from build123d import *

# Parameters (mm, degrees)
SKETCH_W     = 17.5
SKETCH_H     = 16.5
PAD_DEPTH    = 4
SKETCH002_W  = 14.5
SKETCH002_H  = 13.5
POCKET_DEPTH = 5
SKETCH003_W  = 1
SKETCH003_H  = 2.9
PAD001_DEPTH = 3
FILLET_R     = 1
FILLET001_R  = 2
CHAMFER_SIZE = 1


with BuildPart() as part:
    # Sketch → Pad (new body)
    with BuildSketch(Plane.XY):
        Rectangle(SKETCH_W, SKETCH_H)
    extrude(amount=PAD_DEPTH)

    # Sketch002 → Pocket (cut)
    with BuildSketch(Plane.XY.offset(3)):
        Rectangle(SKETCH002_W, SKETCH002_H)
    extrude(amount=POCKET_DEPTH, mode=Mode.SUBTRACT)

    # Sketch003 (on Face11 of Pocket) → Pad001 (join)
    with BuildSketch(Plane.XY.offset(3)):
        with Locations((-2.75, 0)):
            Rectangle(SKETCH003_W, SKETCH003_H)
        with Locations((2.75, 0)):
            Rectangle(SKETCH003_W, SKETCH003_H)
    extrude(amount=PAD001_DEPTH)

    # Fillet
    fillet_edges = [part.edges().sort_by_distance(p)[0] for p in [
        (2.75, 1.45, 3),
        (3.25, 0, 3),
        (2.75, -1.45, 3),
        (2.25, 0, 3),
        (-2.75, 1.45, 3),
        (-3.25, 0, 3),
        (-2.75, -1.45, 3),
        (-2.25, 0, 3),
    ]]
    fillet(fillet_edges, radius=FILLET_R)

    # Fillet001
    fillet001_edges = [part.edges().sort_by_distance(p)[0] for p in [
        (-8.75, 8.25, 2),
        (8.75, 8.25, 2),
        (8.75, -8.25, 2),
        (-8.75, -8.25, 2),
    ]]
    fillet(fillet001_edges, radius=FILLET001_R)

    # Chamfer
    chamfer_edges = [part.edges().sort_by_distance(p)[0] for p in [
        (-8.75, 0, 0),
        (-8.164214, 7.664214, 0),
        (-8.164214, -7.664214, 0),
        (0, 8.25, 0),
        (0, -8.25, 0),
        (8.164214, 7.664214, 0),
        (8.164214, -7.664214, 0),
        (8.75, 0, 0),
    ]]
    chamfer(chamfer_edges, length=CHAMFER_SIZE)


solid = part.part
CAD build for the part. Positions are in the model's coordinates, mm. A direction names the side the tool comes from. Round coordinates to 2 decimals unless told otherwise and drop trailing zeros. Write each loop counter-clockwise with the first axis right and the second up, starting at its lowest first coordinate (ties: lowest second). Pieces come first, ordered by that corner, then holes. Notation, with made-up numbers: M -4,84.25 L 49,84.25 A22 ccw 49,119.25 Z; hole C 4.5,-10.75 d5. An arc over 180 degrees is marked long. Put each result on its own line as item: value. Start each with the question number.
1) Saw through at A-A, the plane x = -0.75. Write the cut outline in (y, z), and give its area (3 significant figures).
2) Saw through at D-D, the plane y = -2.75. Write the cut outline in (x, z), and give its area (3 significant figures).
3) Pull direction Y, two halves, no side cores. Call faces 1 (the flat face through (2.25, 0, 5)), 2 (the cylindrical face through (2.77, 1.89, 3.17)), 3 (the flat face through (-0.09, 7.74, 0.49)): pulls with the +Y half, pulls with the -Y half, needs draft (parallel to the pull), parting line crosses it, or undercut.
4) Saw through at C-C, the plane x = 3. Write the cut outline in (y, z).
5) Pin check, flat tips, straight feed: pin 1 Ø1 at (y, z) = (0.5, 5) entering from -X; pin 2 Ø0.8 at (x, z) = (3, 5) entering from -Y; pin 3 Ø1 at (y, z) = (0, 5.5) entering from +X. Stop position of each tip, or through.
6) Saw through at B-B, the plane y = 0.25. Write the cut outline in (x, z).
7) 3-axis set-ups, long thin cutter, end or side, ignore diameter. For faces 4 (the flat face through (-3, 1.45, 5)), 5 (the flat face through (3, -1.45, 5)), 6 (the conical face through (7.716, 7.238, 0.382)), 7 (the cylindrical face through (-2.73, 1.89, 3.17)), 8 (the flat face through (-2.25, 0, 5)): which of +Z, -Z, +X, -X, +Y, -Y reach the whole face in a straight line?
8) Drill centre lines: probe 1 along Y at (x, z) = (-3, 3.9); probe 2 along Y at (x, z) = (-0.5, 3.6); probe 3 along Z at (x, y) = (5.25, 5.75). Where is each one in solid material? Low to high. Write a range as [from, to].
Resolved:
1. outline: M -8.25,1 L -7.25,0 L 7.25,0 L 8.25,1 L 8.25,4 L 6.75,4 L 6.75,3 L -6.75,3 L -6.75,4 L -8.25,4 Z
1. area: 51.5 mm²
2. outline: M -8.75,1 L -7.75,0 L 7.75,0 L 8.75,1 L 8.75,4 L 7.25,4 L 7.25,3 L -7.25,3 L -7.25,4 L -8.75,4 Z
2. area: 54.5 mm²
3. face 1: needs draft
3. face 2: undercut
3. face 3: pulls with the +Y half
4. outline: M -8.25,1 L -7.25,0 L 7.25,0 L 8.25,1 L 8.25,4 L 6.75,4 L 6.75,3 L 2.45,3 A1 cw 1.45,4 L 1.45,6 L -1.45,6 L -1.45,4 A1 cw -2.45,3 L -6.75,3 L -6.75,4 L -8.25,4 Z
5. pin 1: x = -3.25
5. pin 2: y = -1.45
5. pin 3: x = 3.25
6. outline: M -8.75,1 L -7.75,0 L 7.75,0 L 8.75,1 L 8.75,4 L 7.25,4 L 7.25,3 L 4.25,3 A1 cw 3.25,4 L 3.25,6 L 2.25,6 L 2.25,4 A1 cw 1.25,3 L -1.25,3 A1 cw -2.25,4 L -2.25,6 L -3.25,6 L -3.25,4 A1 cw -4.25,3 L -7.25,3 L -7.25,4 L -8.75,4 Z
7. face 4: +Z, +X, -X, +Y
7. face 5: +Z, +X, -X, -Y
7. face 6: -Z, +X, +Y
7. face 7: +Z
7. face 8: +Z, +Y, -Y
8. probe 1: [-8.25, -6.75], [-1.46, 1.46], [6.75, 8.25]
8. probe 2: [-8.25, -6.75], [6.75, 8.25]
8. probe 3: [0, 3]
